CAD build for the part. Positions are in the model's coordinates, mm. A direction names the side the tool comes from. Round coordinates to 2 decimals unless told otherwise and drop trailing zeros. Loops run counter-clockwise (first coordinate to the right, second up) from the corner with the lowest first, then second, coordinate; pieces in that order, holes last. Notation, with made-up numbers: (18.5, 47.25) -> (70.5, 47.25) arc R20 ccw to (70.5, 72.25) -> close; hole circle Ø2 at (25.5, 12.5). An arc over 180 degrees is marked (long way). Answer as CSV lines item,"result".
```python
from build123d import *

# Parameters (mm, degrees)
F0_W          = 10
F0_H          = 150
F0_W_2        = 15
F0_H_2        = 31
F1_DEPTH      = 5
F2_DEPTH      = 25
F3_DEPTH      = 25
F5_DEPTH      = 25
F5_DEPTH_BACK = 5
F7_DEPTH      = 100


# Not quite as in the source:
# - a feature names something its author has since deleted; it is built from what else it names


with BuildPart() as f1:
    # F0 (on Top) → F1 (new body)
    with BuildSketch(Plane.XY):
        with BuildLine():
            Line((-70.3635856962, -3.0238344104), (-87.8635856962, -3.0238344104))
            Line((-87.8635856962, -3.0238344104), (-87.8635856962, -53.0238344104))
            Line((-87.8635856962, -53.0238344104), (-72.8635856962, -53.0238344104))
            Line((-72.8635856962, -53.0238344104), (-62.8635856962, -53.0238344104))
            Line((-62.8635856962, -53.0238344104), (-52.8635856962, -53.0238344104))
            Line((-52.8635856962, -53.0238344104), (-52.0057213199, -53.0238344104))
            Line((-52.0057213199, -53.0238344104), (-37.8635856962, -38.8816987866))
            Line((-37.8635856962, -38.8816987866), (-37.8635856962, -3.0238344104))
            Line((-37.8635856962, -3.0238344104), (-55.3635856962, -3.0238344104))
            Line((-55.3635856962, -3.0238344104), (-55.3635856962, -12.2124461095))
            ThreePointArc((-55.3635856962, -12.2124461095), (-48.0733862384, -18.6696909434), (-45.3635856962, -28.0238344104))
            ThreePointArc((-45.3635856962, -28.0238344104), (-72.2177291631, -42.8140338681), (-70.3635856962, -12.2124461095))
            Line((-70.3635856962, -12.2124461095), (-70.3635856962, -3.0238344104))
        make_face()
        with Locations((-67.8635856962, -128.0238344104)):
            Rectangle(F0_W, F0_H)
        with Locations((-57.8635856962, -128.0238344104)):
            Rectangle(F0_W, F0_H)
        Polygon((-37.8635856962, -53.0238344104), (-37.8635856962, -38.8816987866), (-52.0057213199, -53.0238344104), align=None)
        Polygon((75.2734992937, -152.0187837765), (-37.8635856962, -38.8816987866), (-37.8635856962, -53.0238344104), (-52.0057213199, -53.0238344104), (61.13136367, -166.1609194002), align=None)
        Polygon((-92.8635856962, -3.0238344104), (-87.8635856962, -3.0238344104), (-70.3635856962, -3.0238344104), (-70.3635856962, 27.9761655896), (-55.3635856962, 27.9761655896), (-55.3635856962, -3.0238344104), (-37.8635856962, -3.0238344104), (-32.8635856962, -3.0238344104), (-32.8635856962, 36.9761655896), (-92.8635856962, 36.9761655896), align=None)
        with Locations((-62.8635856962, 12.4761655896)):
            Rectangle(F0_W_2, F0_H_2)
        with BuildLine():
            Line((-55.3635856962, -3.0238344104), (-70.3635856962, -3.0238344104))
            Line((-70.3635856962, -3.0238344104), (-70.3635856962, -12.2124461095))
            ThreePointArc((-70.3635856962, -12.2124461095), (-62.8635856962, -10.5238344104), (-55.3635856962, -12.2124461095))
            Line((-55.3635856962, -12.2124461095), (-55.3635856962, -3.0238344104))
        make_face()
        with BuildLine():
            ThreePointArc((-55.3635856962, -12.2124461095), (-62.8635856962, -10.5238344104), (-70.3635856962, -12.2124461095))
            Line((-70.3635856962, -12.2124461095), (-70.3635856962, -34.0238344104))
            Line((-70.3635856962, -34.0238344104), (-55.3635856962, -34.0238344104))
            Line((-55.3635856962, -34.0238344104), (-55.3635856962, -12.2124461095))
        make_face()
    extrude(amount=F1_DEPTH)

    # F0 (on Top) → F2 (join)
    with BuildSketch(Plane.XY):
        with BuildLine():
            Line((-70.3635856962, -34.0238344104), (-70.3635856962, -12.2124461095))
            ThreePointArc((-70.3635856962, -12.2124461095), (-72.2177291631, -42.8140338681), (-45.3635856962, -28.0238344104))
            ThreePointArc((-45.3635856962, -28.0238344104), (-48.0733862384, -18.6696909434), (-55.3635856962, -12.2124461095))
            Line((-55.3635856962, -12.2124461095), (-55.3635856962, -34.0238344104))
            Line((-55.3635856962, -34.0238344104), (-70.3635856962, -34.0238344104))
        make_face()
    extrude(amount=F2_DEPTH)

    # F0 (on Top) → F3 (join)
    with BuildSketch(Plane.XY):
        Polygon((-62.8635856962, -203.0238344104), (-72.8635856962, -203.0238344104), (-112.8635856962, -203.0238344104), (-112.8635856962, -223.0238344104), (-12.8635856962, -223.0238344104), (-12.8635856962, -203.0238344104), (-52.8635856962, -203.0238344104), align=None)
    extrude(amount=F3_DEPTH)

    # F4 (on face) → F5 (join, two sides)
    with BuildSketch(Plane(origin=(-38.3726422414, -38.3726422414, 0), x_dir=(-0.7071067812, 0.7071067812, 0), z_dir=(0.7071067812, 0.7071067812, 0))) as f5_sk:
        Polygon((-160.7199146703, 35), (-160.7199146703, 5), (-130.7199146703, 5), align=None)
    extrude(amount=-F5_DEPTH)
    extrude(f5_sk.sketch, amount=F5_DEPTH_BACK)

    # F6 (on face) → F7 (cut, through all)
    with BuildSketch(Plane(origin=(-112.8635856962, 0, 0), x_dir=(0, -1, 0), z_dir=(-1, 0, 0))):
        Polygon((223.0238344104, 25), (208.0238344104, 25), (223.0238344104, 5), align=None)
    extrude(amount=-F7_DEPTH, mode=Mode.SUBTRACT)


solid = f1.part
```
Q1. Slice it at D-D, the plane x = -67. Give the cut face in (y, z), and give its area (3 significant figures).
Results:
outline,"(-223.02, 0) -> (36.98, 0) -> (36.98, 5) -> (-34.02, 5) -> (-34.02, 25) -> (-45.03, 25) -> (-45.03, 5) -> (-203.02, 5) -> (-203.02, 25) -> (-208.02, 25) -> (-223.02, 5) -> close"
area,"1,770 mm2"
Q2. Slice it at B-B, the plane x = -26.5. Give the cut face in (y, z), and give its area (3 significant figures).
Results:
outline,"(-223.02, 0) -> (-203.02, 0) -> (-203.02, 25) -> (-208.02, 25) -> (-223.02, 5) -> close; (-78.53, 0) -> (-50.25, 0) -> (-50.25, 5) -> (-78.53, 5) -> close"
area,"491 mm2"
Q3. Slice it at C-C, the plane y = -96. Give the cut face in (x, z), and give its area (3 significant figures).
Results:
outline,"(-72.86, 0) -> (-52.86, 0) -> (-52.86, 5) -> (-72.86, 5) -> close; (-9.03, 0) -> (19.25, 0) -> (19.25, 5) -> (-9.03, 5) -> close"
area,"241 mm2"
Q4. Probe L1, parallel to Z at x = -61, y = -165.5; L2, parallel to X at y = -212, z = 11; L3, parallel to X at y = -146.5, z = 28.5. List the from-to ranges inside material, lowest first. Write a range as [from, to].
Results:
L1,"[0, 5]"
L2,"[-112.86, -12.86]"
L3,"[71.6, 76.83]"
Q5. Two-plate mould, pull along X, no slides. Class faces 1 (the flat face through (-87.864, -28, 2)), 2 (the flat face through (-63, -36, 25)), 3 (the flat face through (-52.864, -129, 2)): pulls with the +X half, pulls with the -X half, needs draft (parallel to the pull), parting line crosses it, or undercut.
Results:
face 1,"pulls with the -X half"
face 2,"needs draft"
face 3,"undercut"
Q6. Tool access for faces 4 (the flat face through (-63, -34.024, 15)), 5 (the flat face through (-92.864, 17, 2)), 6 (the flat face through (-72.864, -129, 2)), 7 (the flat face through (3.77, -108.8, 2.46)), 8 (the flat face through (-35, -3.024, 2)): list every direction of +Z, -Z, +X, -X, +Y, -Y with a clear straight run to the whole face (end or side of a thin tool).
Results:
face 4,"+Z, +Y"
face 5,"+Z, -Z, -X, +Y"
face 6,"+Z, -Z, -X"
face 7,"-Z"
face 8,"+Z, -Z, +X"
Q7. Drop flat-ended pins along their axis: pin 1 Ø4 at (y, z) = (12.5, 1.5) entering from +X; pin 2 Ø1.5 at (y, z) = (-114, 3) entering from +X; pin 3 Ø6 at (x, z) = (-40.5, 18) entering from +Y. Give the stop position or say it passes through.
Results:
pin 1,"x = -32.86"
pin 2,"x = 38"
pin 3,"y = -203.02"
Q8. Slice it at A-A, the plane z = 13.5. Give the cut face in (x, y), and give its area (3 significant figures).
Results:
outline,"(-112.86, -216.65) -> (-12.86, -216.65) -> (-12.86, -203.02) -> (-112.86, -203.02) -> close; (-70.36, -34.02) -> (-70.36, -12.21) arc R17.5 ccw (long way) to (-55.36, -12.21) -> (-55.36, -34.02) -> close; (42.39, -154.49) -> (57.6, -169.7) -> (78.81, -148.48) -> (63.61, -133.28) -> close"
area,"2,630 mm2"
